Geometry: see drawing. Coordinates: mm, zero at the bounding-box minimum. Give positions to 0.01 mm unless a question says otherwise; leave off trailing zeros. Write each loop counter-clockwise with the first axis right and the second up, starting at its lowest first coordinate (ties: lowest second). Pieces come first, ordered by that corner, then holes. Notation, with made-up numbers: (85.25, -27) -> (95.25, -27) arc R10 ccw to (95.25, -18) -> close; hole circle Ø11 at (85, -12). An arc over 180 degrees is marked (long way). Use CSV: the item, a comma, the result in double quotes. Start each with the question number.
1) Section A-A (x = 75). Output: boundary loops of the cut face in (y, z).
2) Section B-B (y = 15). Output: boundary loops of the cut face in (x, z).
3) Contact query for a flat-ended pin moving along its axis: P1, Ø6, axis at x = 45, y = 15, coming from the -Z side. Output: stop coordinate, or through.
4) Material intervals for line 1 (Y direction, x = 15, z = 1.45); line 2 (X direction, y = 78, z = 1.75); line 3 (X direction, y = 43, z = 0.45), sorted ascending. Write a range as [from, to].
5) Section D-D (z = 0.45). Output: boundary loops of the cut face in (x, y), plus the area to 3 significant figures.
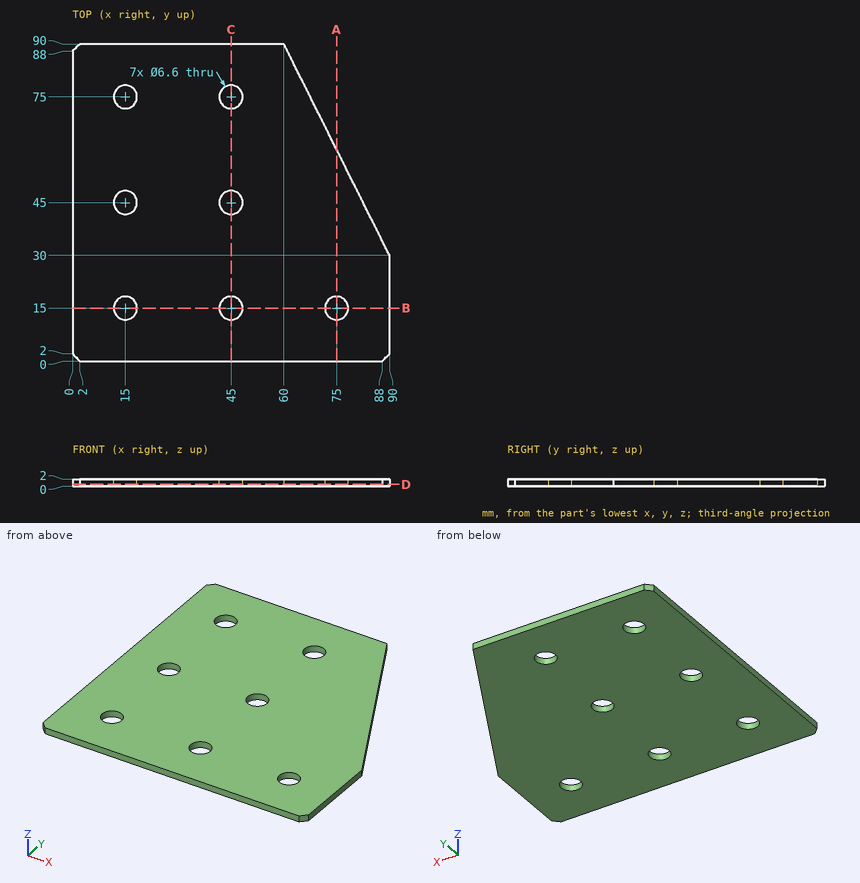
Answers follow:
1,outline,"(0, 0) -> (11.7, 0) -> (11.7, 2) -> (0, 2) -> close; (18.3, 0) -> (60, 0) -> (60, 2) -> (18.3, 2) -> close"
2,outline,"(0, 0) -> (11.7, 0) -> (11.7, 2) -> (0, 2) -> close; (18.3, 0) -> (41.7, 0) -> (41.7, 2) -> (18.3, 2) -> close; (48.3, 0) -> (71.7, 0) -> (71.7, 2) -> (48.3, 2) -> close; (78.3, 0) -> (90, 0) -> (90, 2) -> (78.3, 2) -> close"
3,P1,"passes through"
4,line 1,"y = [0, 11.7], [18.3, 41.7], [48.3, 71.7], [78.3, 90]"
4,line 2,"x = [0, 13.63], [16.37, 43.63], [46.37, 66]"
4,line 3,"x = [0, 12.38], [17.62, 42.38], [47.62, 83.5]"
5,outline,"(0, 2) -> (2, 0) -> (88, 0) -> (90, 2) -> (90, 30) -> (60, 90) -> (2, 90) -> (0, 88) -> close; hole circle Ø6.6 at (15, 15); hole circle Ø6.6 at (15, 45); hole circle Ø6.6 at (15, 75); hole circle Ø6.6 at (45, 15); hole circle Ø6.6 at (45, 45); hole circle Ø6.6 at (45, 75); hole circle Ø6.6 at (75, 15)"
5,area,"6,950 mm^2"
